```python
from build123d import *

# Parameters (mm, degrees)
MODEL_W             = 10.99999994
MODEL_H             = 5.349999293
MODEL_W_2           = 5.350001157
MODEL_H_2           = 10.000001639
MODEL_H_3           = 9.999997913
MODEL_H_4           = 10.000005364
MODEL_H_5           = 9.999990463
MODEL_W_3           = 19.999999553
MODEL_H_6           = 5.350001156
MODEL_H_7           = 5.349993706
MODEL_H_8           = 5.350008607
MODEL_W_4           = 5.350001156
MODEL_H_9           = 8.999999612
MODEL_W_5           = 5.350004882
MODEL_H_10          = 12.000000104
MODEL_W_6           = 19.999988377
MODEL_W_7           = 19.999995828
MODEL_H_11          = 5.349999992
MODEL_H_12          = 11.999994516
MODEL_W_8           = 10.999999941
BOSS_EXTRUDE1_DEPTH = 5.35


with BuildPart() as part:
    # Model → Boss-Extrude1 (new body)
    with BuildSketch(Plane.XY):
        with BuildLine():
            Line((295.349999331, 304.108172655), (295.349999331, 265.608172864))
            Line((295.349999331, 265.608172864), (300.699999556, 265.608172864))
            Line((300.699999556, 265.608172864), (300.699999556, 218.941502273))
            Line((300.699999556, 218.941502273), (295.349999331, 218.941502273))
            Line((295.349999331, 218.941502273), (295.349999331, 180.441506207))
            Line((295.349999331, 180.441506207), (300.699999556, 180.441506207))
            Line((300.699999556, 180.441506207), (300.699999556, 133.774831891))
            Line((300.699999556, 133.774831891), (295.349999331, 133.774831891))
            Line((295.349999331, 133.774831891), (295.349999331, 95.274835825))
            Line((295.349999331, 95.274835825), (300.699999556, 95.274835825))
            Line((300.699999556, 95.274835825), (300.699999556, 48.608183861))
            Line((300.699999556, 48.608183861), (295.349999331, 48.608183861))
            Line((295.349999331, 48.608183861), (295.349999331, 10.108172894))
            Line((295.349999331, 10.108172894), (275.349999778, 10.108172894))
            Line((275.349999778, 10.108172894), (275.349999778, 15.458166599))
            Line((275.349999778, 15.458166599), (255.350000225, 15.458166599))
            Line((255.350000225, 15.458166599), (255.350000225, 0))
            Line((255.350000225, 0), (45.349999331, 0))
            Line((45.349999331, 0), (45.349999331, 15.458166599))
            Line((45.349999331, 15.458166599), (25.349999778, 15.458166599))
            Line((25.349999778, 15.458166599), (25.349999778, 10.108172894))
            Line((25.349999778, 10.108172894), (5.350000225, 10.108172894))
            Line((5.350000225, 10.108172894), (5.350000225, 48.608183861))
            Line((5.350000225, 48.608183861), (0, 48.608183861))
            Line((0, 48.608183861), (0, 95.274835825))
            Line((0, 95.274835825), (5.350000225, 95.274835825))
            Line((5.350000225, 95.274835825), (5.350000225, 133.774831891))
            Line((5.350000225, 133.774831891), (0, 133.774831891))
            Line((0, 133.774831891), (0, 180.441506207))
            Line((0, 180.441506207), (5.350000225, 180.441506207))
            Line((5.350000225, 180.441506207), (5.350000225, 218.941502273))
            Line((5.350000225, 218.941502273), (0, 218.941502273))
            Line((0, 218.941502273), (0, 265.608172864))
            Line((0, 265.608172864), (5.350000225, 265.608172864))
            Line((5.350000225, 265.608172864), (5.350000225, 304.108172655))
            Line((5.350000225, 304.108172655), (25.349999778, 304.108172655))
            Line((25.349999778, 304.108172655), (25.349999778, 298.75817243))
            Line((25.349999778, 298.75817243), (45.349999331, 298.75817243))
            Line((45.349999331, 298.75817243), (45.349999331, 304.108172655))
            ThreePointArc((45.349999331, 304.108172655), (52.670508573, 311.428680858), (55.35000097, 321.428681677))
            Line((55.35000097, 321.428681677), (55.35000097, 329.108174443))
            ThreePointArc((55.35000097, 329.108174443), (61.207865188, 343.250309909), (75.350000523, 349.108174443))
            Line((75.350000523, 349.108174443), (225.349999033, 349.108174443))
            ThreePointArc((225.349999033, 349.108174443), (239.492134368, 343.250309909), (245.349998586, 329.108174443))
            Line((245.349998586, 329.108174443), (245.349998586, 321.428681677))
            ThreePointArc((245.349998586, 321.428681677), (248.029490983, 311.428680858), (255.350000225, 304.108172655))
            Line((255.350000225, 304.108172655), (255.350000225, 298.75817243))
            Line((255.350000225, 298.75817243), (275.349999778, 298.75817243))
            Line((275.349999778, 298.75817243), (275.349999778, 304.108172655))
            Line((275.349999778, 304.108172655), (295.349999331, 304.108172655))
        make_face()
        with Locations((223.849999718, 336.625010707)):
            Rectangle(MODEL_W, MODEL_H, mode=Mode.SUBTRACT)
        with Locations((184.850002639, 336.625010707)):
            Rectangle(MODEL_W, MODEL_H, mode=Mode.SUBTRACT)
        with Locations((108.025002294, 263.726172969)):
            Rectangle(MODEL_W_2, MODEL_H_2, mode=Mode.SUBTRACT)
        with Locations((108.025002294, 192.647505552)):
            Rectangle(MODEL_W_2, MODEL_H_3, mode=Mode.SUBTRACT)
        with Locations((108.025002294, 121.568836272)):
            Rectangle(MODEL_W_2, MODEL_H_4, mode=Mode.SUBTRACT)
        with Locations((108.025002294, 50.490170718)):
            Rectangle(MODEL_W_2, MODEL_H_5, mode=Mode.SUBTRACT)
        with Locations((35.349999555, 228.186842054)):
            Rectangle(MODEL_W_3, MODEL_H_6, mode=Mode.SUBTRACT)
        with Locations((35.349999555, 157.108172774)):
            Rectangle(MODEL_W_3, MODEL_H_7, mode=Mode.SUBTRACT)
        with Locations((35.349999555, 86.02950722)):
            Rectangle(MODEL_W_3, MODEL_H_8, mode=Mode.SUBTRACT)
        with Locations((105.524997227, 320.450009778)):
            Rectangle(MODEL_W_4, MODEL_H_9, mode=Mode.SUBTRACT)
        with Locations((68.025001325, 288.600009866)):
            Rectangle(MODEL_W_5, MODEL_H_10, mode=Mode.SUBTRACT)
        with Locations((150.349999777, 8.675009012)):
            Rectangle(MODEL_W_6, MODEL_H_7, mode=Mode.SUBTRACT)
        with Locations((200.350000523, 8.675009012)):
            Rectangle(MODEL_W_7, MODEL_H_7, mode=Mode.SUBTRACT)
        with Locations((100.349999033, 304.275010363)):
            Rectangle(MODEL_W_7, MODEL_H_11, mode=Mode.SUBTRACT)
        with Locations((150.349999777, 304.275010363)):
            Rectangle(MODEL_W_6, MODEL_H_11, mode=Mode.SUBTRACT)
        with Locations((232.674998231, 24.350002408)):
            Rectangle(MODEL_W_5, MODEL_H_12, mode=Mode.SUBTRACT)
        with Locations((68.025001325, 24.350002408)):
            Rectangle(MODEL_W_5, MODEL_H_12, mode=Mode.SUBTRACT)
        with Locations((100.349999033, 8.675009012)):
            Rectangle(MODEL_W_7, MODEL_H_7, mode=Mode.SUBTRACT)
        with Locations((200.350000523, 304.275010363)):
            Rectangle(MODEL_W_7, MODEL_H_11, mode=Mode.SUBTRACT)
        with Locations((232.674998231, 288.600009866)):
            Rectangle(MODEL_W_5, MODEL_H_10, mode=Mode.SUBTRACT)
        with Locations((115.849996917, 336.625010707)):
            Rectangle(MODEL_W, MODEL_H, mode=Mode.SUBTRACT)
        with Locations((76.849999838, 336.625010707)):
            Rectangle(MODEL_W_8, MODEL_H, mode=Mode.SUBTRACT)
        with Locations((195.175002329, 320.450009778)):
            Rectangle(MODEL_W_4, MODEL_H_9, mode=Mode.SUBTRACT)
        with Locations((265.350000002, 86.02950722)):
            Rectangle(MODEL_W_3, MODEL_H_8, mode=Mode.SUBTRACT)
        with Locations((265.350000002, 157.108172774)):
            Rectangle(MODEL_W_3, MODEL_H_7, mode=Mode.SUBTRACT)
        with Locations((265.350000002, 228.186842054)):
            Rectangle(MODEL_W_3, MODEL_H_6, mode=Mode.SUBTRACT)
        with Locations((192.674997263, 50.490170718)):
            Rectangle(MODEL_W_2, MODEL_H_5, mode=Mode.SUBTRACT)
        with Locations((192.674997263, 121.568836272)):
            Rectangle(MODEL_W_2, MODEL_H_4, mode=Mode.SUBTRACT)
        with Locations((192.674997263, 192.647505552)):
            Rectangle(MODEL_W_2, MODEL_H_3, mode=Mode.SUBTRACT)
        with Locations((192.674997263, 263.726172969)):
            Rectangle(MODEL_W_2, MODEL_H_2, mode=Mode.SUBTRACT)
    extrude(amount=BOSS_EXTRUDE1_DEPTH)


solid = part.part
```
For this review, take the finished solid that the model builds, in its own axes (mm). Round coordinates to 2 decimals unless told otherwise and drop trailing zeros. Write each loop counter-clockwise with the first axis right and the second up, starting at its lowest first coordinate (ties: lowest second). Pieces come first, ordered by that corner, then holes. Notation, with made-up numbers: (48, 44.5) - (67, 44.5) arc R22 ccw to (67, 56.5) - close; hole circle Ø8 at (60.5, -30). An arc over 180 degrees is marked (long way). Answer as a JSON object with one key per item and string values.
1. We need section A-A on y = 122.5. Give the boundary of the cut face in (x, z).
Response values:
{"outline": "(5.35, 0) - (105.35, 0) - (105.35, 5.35) - (5.35, 5.35) - close; (110.7, 0) - (190, 0) - (190, 5.35) - (110.7, 5.35) - close; (195.35, 0) - (295.35, 0) - (295.35, 5.35) - (195.35, 5.35) - close"}
2. We need section B-B on x = 147. Give the boundary of the cut face in (y, z).
Response values:
{"outline": "(0, 0) - (6, 0) - (6, 5.35) - (0, 5.35) - close; (11.35, 0) - (301.6, 0) - (301.6, 5.35) - (11.35, 5.35) - close; (306.95, 0) - (349.11, 0) - (349.11, 5.35) - (306.95, 5.35) - close"}
3. We need section D-D on z = 2.4. Count the separate pieces of the cut face and the enclosed holes in it, then the cut area to 3 significant figures.
Response values:
{"separate pieces": "1", "enclosed holes": "30", "area": "94,600 mm2"}
4. For pin 1 Ø10 at (x, y) = (242.5, 249.5) entering from -Z; pin 2 Ø2.5 at (x, z) = (38.5, 2) entering from -Y; pin 3 Ø1.6 at (y, z) = (335.5, 2) entering from +X; pin 4 Ø2.5 at (x, z) = (297, 2) entering from +Y, all flat-tipped, find the tip position at first contact; note any pin that passes through.
Response values:
{"pin 1": "stops at z = 0", "pin 2": "stops at y = 15.46", "pin 3": "stops at x = 244.55", "pin 4": "stops at y = 265.61"}
5. To check wall thickness, follow line 1 along X through (y, z) = (191, 5.05); line 2 along Y through (x, z) = (96, 1.75); line 3 along X through (y, z) = (25.5, 2.2). State the ranges of each line that lie inside material, in increasing order.
Response values:
{"line 1": "x = 5.35 to 105.35, 110.7 to 190, 195.35 to 295.35", "line 2": "y = 0 to 6, 11.35 to 301.6, 306.95 to 349.11", "line 3": "x = 5.35 to 65.35, 70.7 to 230, 235.35 to 295.35"}
6. We need section C-C on x = 116.5. Give the boundary of the cut face in (y, z), then the cut area to 3 significant figures.
Response values:
{"outline": "(0, 0) - (333.95, 0) - (333.95, 5.35) - (0, 5.35) - close; (339.3, 0) - (349.11, 0) - (349.11, 5.35) - (339.3, 5.35) - close", "area": "1,840 mm2"}
